Model file for the job. Use its own axes, mm. Face numbers are marked on the shaded views. A direction names the side the tool comes from. Give positions to 0.01 mm unless a question says otherwise; leave off trailing zeros. Loops run counter-clockwise (first coordinate to the right, second up) from the corner with the lowest first, then second, coordinate; pieces in that order, holes last. Notation, with made-up numbers: (10.25, -17.75) - (26.25, -17.75) arc R9 cw to (26.25, -13.75) - close; hole circle Ø8 at (69.5, 28.5). An arc over 180 degrees is marked (long way). Answer as CSV lines item,"result". Start each with the question number.
Item 1: Tool access for the marked faces 1, 2, 3, 4 and 5: list every direction of +Z, -Z, +X, -X, +Y, -Y with a clear straight run to the whole face (end or side of a thin tool).
Item 2: Saw through at B-B on z = 7. State how many separate pieces and enclosed holes the cut face has, plus the area to 3 significant figures.
Item 3: Drill centre lines: L1, parallel to Y at x = -26.37, z = 4.5; L2, parallel to Y at x = 19.27, z = 6.75; L3, parallel to Y at x = 16.5, z = 7.25. Where is each one in solid material? Low to high. Write a range as from..to.
Item 4: Saw through at A-A on z = 1.25. Give the cut face in (x, y).
Item 5: Pin check, flat tips, straight feed: pin 1 (3 mm diameter, centred on y = 6.5, z = 2, fed in from -X); pin 2 (3 mm diameter, centred on x = 19.27, y = -5.2, fed in from +Z); pin 3 (4 mm diameter, centred on y = -6, z = 6.5, fed in from -X); pin 4 (5.5 mm diameter, centred on x = 13.5, z = 6.5, fed in from -Y). Stop position of each tip, or through.
from build123d import *

# Parameters (mm, degrees)
F1_DEPTH    = 10
F2_W        = 10.0960650777
F2_H        = 2.7
F3_DEPTH    = 6
F4_R        = 5
F5_T1_DEPTH = 21.1923143391
F5_T3_DEPTH = 15.6473434867
F5_T5_DEPTH = 30
F7_DEPTH    = 2


# Not quite as in the source:
# - a fillet or chamfer that OpenCascade refuses, or shapes differently, is made with other operations: its cross-section is extruded or revolved along the edge and cut away or added


with BuildPart() as f1:
    # F0 (on Top) → F1 (new body)
    with BuildSketch(Plane.XY):
        Polygon((30, 9), (0, 9), (0, -1.8), (15, -1.8), (15, -9), (19.5954625243, -9), (30, -2.6151265483), align=None)
        with BuildLine():
            ThreePointArc((21.17, -5.2), (17.9264971157, -6.5435028843), (19.27, -3.3))
            ThreePointArc((19.27, -3.3), (20.6135028843, -3.8564971157), (21.17, -5.2))
        make_face(mode=Mode.SUBTRACT)
        with BuildLine():
            ThreePointArc((19.27, 3.9), (17.9264971157, 7.1435028843), (21.17, 5.8))
            ThreePointArc((21.17, 5.8), (20.6135028843, 4.4564971157), (19.27, 3.9))
        make_face(mode=Mode.SUBTRACT)
        with BuildLine():
            ThreePointArc((24.47, 5.8), (26.37, 7.7), (28.27, 5.8))
            ThreePointArc((28.27, 5.8), (26.37, 3.9), (24.47, 5.8))
        make_face(mode=Mode.SUBTRACT)
    extrude(amount=F1_DEPTH)

    # F2 (on face) → F3 (cut)
    with BuildSketch(Plane.XY.offset(10)):
        with BuildLine():
            ThreePointArc((11.6039349223, 0.3250306588), (9.2827431951, 3.7535073497), (13.3280728534, 4.6353754864))
            Line((13.3280728534, 4.6353754864), (16.2527744297, 1.8499454137))
            ThreePointArc((16.2527744297, 1.8499454137), (16.328577113, 2.3348713274), (16.3539349223, 2.8250306588))
            ThreePointArc((16.3539349223, 2.8250306588), (16.0328522645, 4.5417691876), (15.1130123218, 6.0264172029))
            ThreePointArc((15.1130123218, 6.0264172029), (7.5069370658, 5.2285923001), (10.5215341623, -1.8))
            Line((10.5215341623, -1.8), (12.6863356823, -1.8))
            ThreePointArc((12.6863356823, -1.8), (14.376262754, -1.0320016711), (15.6428085277, 0.3250306588))
            Line((15.6428085277, 0.3250306588), (11.6039349223, 0.3250306588))
        make_face()
        with BuildLine():
            ThreePointArc((16.3539349223, 2.8250306588), (16.328577113, 2.3348713274), (16.2527744297, 1.8499454137))
            Line((16.2527744297, 1.8499454137), (16.9487625085, 1.1870996243))
            ThreePointArc((16.9487625085, 1.1870996243), (17.0635074373, 1.0219903081), (17.1039349223, 0.8250306588))
            ThreePointArc((17.1039349223, 0.8250306588), (16.9574883129, 0.4714772682), (16.6039349223, 0.3250306588))
            Line((16.6039349223, 0.3250306588), (15.6428085277, 0.3250306588))
            ThreePointArc((15.6428085277, 0.3250306588), (14.376262754, -1.0320016711), (12.6863356823, -1.8))
            Line((12.6863356823, -1.8), (15, -1.8))
            Line((15, -1.8), (15, -1.9249693412))
            Line((15, -1.9249693412), (19.9039349223, -1.9249693412))
            Line((19.9039349223, -1.9249693412), (19.9039349223, 0.7750306588))
            Line((19.9039349223, 0.7750306588), (15.1130123218, 6.0264172029))
            ThreePointArc((15.1130123218, 6.0264172029), (16.0328522645, 4.5417691876), (16.3539349223, 2.8250306588))
        make_face()
        with Locations((24.9519674612, -0.5749693412)):
            Rectangle(F2_W, F2_H)
    extrude(amount=-F3_DEPTH, mode=Mode.SUBTRACT)

    # F4
    f4_edges = [f1.edges().sort_by_distance(p)[0] for p in [
        (19.903935, 0.775031, 7),
    ]]
    fillet(f4_edges, radius=F4_R)

    # F5: fillet of radius 4 on 4 edges, made by hand

    # F5_s2 → F5_t1 (cut)
    with BuildSketch(Plane.XY.offset(-5.5961571696)):
        with BuildLine():
            ThreePointArc((30, -0.3766636805), (29.4905957559, -2.3300559271), (28.0921293656, -3.7859150232))
            Line((28.0921293656, -3.7859150232), (30, -2.6151265483))
            Line((30, -2.6151265483), (30, -0.3766636805))
        make_face()
    extrude(amount=F5_T1_DEPTH, mode=Mode.SUBTRACT)

    # F5_s4 → F5_t3 (cut)
    with BuildSketch(Plane.XY.offset(-2.8236717433)):
        with BuildLine():
            ThreePointArc((20.5581231925, -8.4092513427), (19.5529608525, -8.8494808332), (18.465993827, -9))
            Line((18.465993827, -9), (19.5954625243, -9))
            Line((19.5954625243, -9), (20.5581231925, -8.4092513427))
        make_face()
    extrude(amount=F5_T3_DEPTH, mode=Mode.SUBTRACT)

    # F5_s6 → F5_t5 (cut)
    with BuildSketch(Plane.XY.offset(-10)):
        with BuildLine():
            ThreePointArc((15, -5), (16.1715728753, -7.8284271247), (19, -9))
            Line((19, -9), (15, -9))
            Line((15, -9), (15, -5))
        make_face()
        with BuildLine():
            ThreePointArc((30, 5), (28.8284271247, 7.8284271247), (26, 9))
            Line((26, 9), (30, 9))
            Line((30, 9), (30, 5))
        make_face()
    extrude(amount=F5_T5_DEPTH, mode=Mode.SUBTRACT)

    # F6 (on face) → F7 (cut)
    with BuildSketch(Plane.XZ.offset(1.8)):
        Polygon((0, 10), (0, 0), (15, 0), (15, 4), (10.5215341623, 4), (10.5215341623, 10), align=None)
    extrude(amount=-F7_DEPTH, mode=Mode.SUBTRACT)

    # F8: F1 across plane


with BuildPart() as f1_1:
    add(f1.part)
    add(f1.part.mirror(Plane.YZ))


solid = f1_1.part
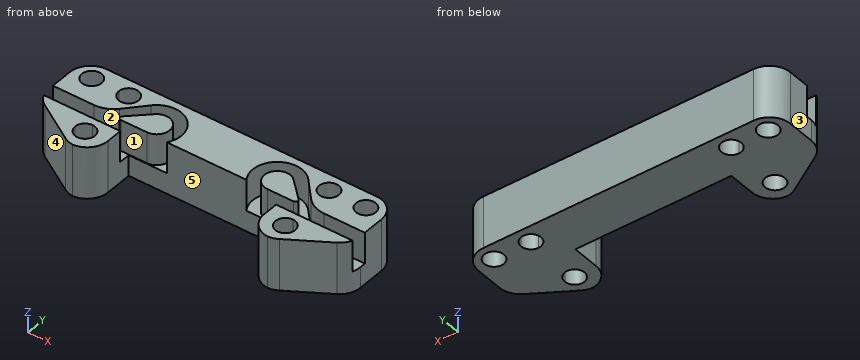
Responses:
1,face 1,"+Z, -X"
1,face 2,"+Z"
1,face 3,"+Z, -Z, -X, +Y, -Y"
1,face 4,"+Z, -Z, -X, -Y"
1,face 5,"+Z, -Z, -Y"
2,separate pieces,"5"
2,enclosed holes,"6"
2,area,"495 mm2"
3,L1,"-4.84..-1.92, 0.78..3.9, 7.7..8.98"
3,L2,"-8.92..-7.1, -3.3..-1.92, 1.66..3.9, 7.7..9"
3,L3,"-8.12..-1.92, 0.33..1.61, 4.51..9"
4,outline,"(-30, -0.38) arc R4 ccw to (-28.09, -3.79) - (-20.56, -8.41) arc R4 ccw to (-18.73, -8.99) arc R4 ccw to (-15, -5) - (-15, 0.2) - (15, 0.2) - (15, -5) arc R4 ccw to (18.73, -8.99) arc R4 ccw to (20.56, -8.41) - (28.09, -3.79) arc R4 ccw to (30, -0.38) - (30, 5) arc R4 ccw to (26, 9) - (-26, 9) arc R4 ccw to (-30, 5) - close; hole circle Ø3.8 at (-26.37, 5.8); hole circle Ø3.8 at (-19.27, -5.2); hole circle Ø3.8 at (-19.27, 5.8); hole circle Ø3.8 at (19.27, -5.2); hole circle Ø3.8 at (19.27, 5.8); hole circle Ø3.8 at (26.37, 5.8)"
5,pin 1,"x = -30"
5,pin 2,"through"
5,pin 3,"x = -27.74"
5,pin 4,"y = -7.9"
